Input: part model. Units: mm. Frame: model coordinates. A direction names the side the tool comes from. Coordinates: 2 decimals unless noted, no trailing zeros. Order: outer loops, then holes, each group sorted by start corner. A loop starts at its lowest first (then second) coordinate and runs counter-clockwise, first axis right, second up.
Autodesk Fusion 360 part; units mm, degrees
sketch "bottom" plane through (0, 0, 0) normal (0, 0, 1) x (1, 0, 0)
  line L0 (-22.5627, 0) -> (-67, 0)
  line L1 (-67, 88) -> (-22.5147, 88)
  circle A0 centre (-36, 69) radius 5
  circle A1 centre (-36, 19) radius 5
  line L2 (13.411, 30.589) -> (-13.3703, 3.8076)
  line L3 (13.435, 57.435) -> (-13.3223, 84.1924)
  line L4 (-67, 88) -> (-80, 88)
  line L5 (-80, 0) -> (-67, 0)
  arc A2 (-13.3223, 84.1924) -> (-22.5147, 88) centre (-22.5147, 75) ccw
  arc A3 (12.6084, 29.7863) -> (13.435, 57.435) centre (0, 44) ccw
  arc A4 (-22.5627, 0) -> (-13.3703, 3.8076) centre (-22.5627, 13) ccw
  line L6 (-64, 49) -> (-60, 49)
  line L7 (-60, 49) -> (-60, 39)
  line L8 (-60, 39) -> (-64, 39)
  circle A5 centre (-86, 44) radius 9.5
  line L9 (-64, 60) -> (-64, 49)
  line L10 (-64, 39) -> (-64, 28)
  arc A6 (-86, 63) -> (-85.9962, 25) centre (-86, 44) ccw
  line L11 (-67, 0) -> (-67, 25)
  line L12 (-67, 63) -> (-67, 88)
  line L13 (-67, 0) -> (-67, 25)
  line L14 (-67, 63) -> (-67, 88)
  arc A7 (-64, 28) -> (-67, 25) centre (-64, 25) ccw
  arc A8 (-67, 63) -> (-64, 60) centre (-64, 63) ccw
  line L15 (-85.9962, 25) -> (-86.0038, 25) construction
  arc A9 (-80, 19) -> (-86, 25) centre (-86, 19) ccw
  line L16 (-80, 19) -> (-80, 0)
  line L17 (-80, 88) -> (-80, 69)
  arc A10 (-86, 63) -> (-80, 69) centre (-86, 69) ccw
  dimension "d1" = 67
  dimension "d3" = 19
  dimension "d4" = 19
  dimension "d5" = 10
  dimension "d6" = 10
  dimension "d15" = 45
  dimension "d16" = 13
  dimension "d17" = 13
  dimension "d18" = 13
  dimension "d20" = 3
  dimension "d21" = 38
  dimension "d23" = 4
  dimension "d24" = 10
  dimension "d25" = 39
  dimension "d26" = 6
  dimension "d27" = 6
  dimension "d30" = 19
  dimension "d31" = 38
  dimension "d38" = 6
  dimension "d39" = 6
extrude "Extrude1" add sketch "bottom" along normal blind 10
extrude "Extrude2" cut sketch "bottom" along normal blind 40 contours L4 L5 L6 L7 L8 L9 L10 A6 L11 L12 L13 L14 A7 A8 A9 L16 L17 A10
extrude "Extrude3" add sketch "bottom" along normal blind 40 contours L4 L5 L6 L7 L8 L9 L10 A6 L11 L12 L13 L14 A7 A8 A9 L16 L17 A10
extrude "Extrude4" add 1 faces at (-71.3333, 73.3333, 40) along direction (0, 0, 1) blind 10
sketch "triangle" plane through (0, 0, 0) normal (0, -1, 0) x (1, 0, 0)
  line L0 (-80, 0) -> (-22.5627, 0)
  line L1 (-22.5627, 0) -> (-22.5627, 10)
  line L2 (-22.5627, 10) -> (-67, 10)
  line L3 (-67, 10) -> (-67, 50)
  line L4 (-67, 50) -> (-80, 50)
  line L5 (-80, 50) -> (-80, 0)
  line L6 (-60, 10) -> (-3, 10)
  line L7 (-60, 10) -> (-60, 50)
  line L8 (-60, 50) -> (-3, 10)
  dimension "d42" = 57
extrude "Extrude5" add sketch "triangle" along normal blind -49 and the other way blind 39 contours L2 L6 L7 L8
Item 1: Access query for faces 4 (the face through (-81.803, 23.288, 24.65)), 5 (the face through (-80, 79, 25)), 6 (the face through (-66.1, 60.86, 29.72)), 7 (the face through (-34, 54, 10)), 8 (the face through (-66.14, 27.1, 29.72)). Directions: +Z, -Z, +X, -X, +Y, -Y. A direction counts if a zero-diameter tool reaches every point of the face in a straight line with its end or side. Return the directions, or none.
Response values:
face 4: +Z, -Z, -X, -Y
face 5: +Z, -Z, -X, +Y
face 6: +Z, +X, +Y
face 7: +Z, +X
face 8: +Z, +X, -Y
Item 2: Cut plane C-C on z = 37. Return loops of the section in (x, y) (3 decimals), then the cut area to 3 significant figures.
Response values:
outline: (-86, 63) arc R19 ccw to (-85.996, 25) arc R6 cw to (-80, 19) - (-80, 0) - (-67, 0) - (-67, 25) arc R3 cw to (-64, 28) - (-64, 39) - (-41.475, 39) - (-41.475, 49) - (-64, 49) - (-64, 60) arc R3 cw to (-67, 63) - (-67, 88) - (-80, 88) - (-80, 69) arc R6 cw to start; hole circle Ø19 at (-86, 44)
area: 2,000 mm2
Item 3: Ray query, probe 1 along Y at (x, z) = (-36, 6.5); probe 2 along Y at (x, z) = (-59.5, 14); probe 3 along Y at (x, z) = (-86, 10.5). Return the intervals inside material, ascending.
Response values:
probe 1: y = 0 to 14, 24 to 64, 74 to 88
probe 2: y = 39 to 49
probe 3: y = 25 to 34.5, 53.5 to 63
Item 4: Draft query along X for faces 1 (the face through (-40, 66, 5)), 2 (the face through (-73, 45, 50)), 3 (the face through (-31.9, 43.93, 30.28)). Return one class per face: pulls with the +X half, pulls with the -X half, needs draft (parallel to the pull), parting line crosses it, or undercut.
Response values:
face 1: undercut
face 2: needs draft
face 3: pulls with the +X half
Item 5: Cut plane B-B on z = 8.5. Return loops of the section in (x, y) (3 decimals).
Response values:
outline: (-86, 63) arc R19 ccw to (-85.996, 25) arc R6 cw to (-80, 19) - (-80, 0) - (-22.563, 0) arc R13 ccw to (-13.37, 3.808) - (12.608, 29.786) arc R19 ccw to (13.435, 57.435) - (-13.322, 84.192) arc R13 ccw to (-22.515, 88) - (-80, 88) - (-80, 69) arc R6 cw to start; hole circle Ø19 at (-86, 44); hole circle Ø10 at (-36, 19); hole circle Ø10 at (-36, 69)
Item 6: Cut plane A-A on y = 44. Return loops of the section in (x, z).
Response values:
outline: (-105, 0) - (-95.5, 0) - (-95.5, 50) - (-105, 50) - close; (-76.5, 0) - (19, 0) - (19, 10) - (-3, 10) - (-60, 50) - (-76.5, 50) - close
Item 7: Cut plane D-D on x = 1.5. Return loops of the section in (y, z), then the cut area to 3 significant figures.
Response values:
outline: (18.68, 0) - (69.37, 0) - (69.37, 10) - (18.68, 10) - close
area: 507 mm2
Item 8: Pin query (flat end, axial travel): pin 1 Ø2 at (y, z) = (43, 40.5) entering from +X; pin 2 Ø7.5 at (y, z) = (13.5, 39) entering from +X; pin 3 Ø10 at (y, z) = (40.5, 30) entering from +X (3 decimals). Return the tip coordinate at first contact, or that it passes through.
Response values:
pin 1: stops at x = -45.04
pin 2: stops at x = -67
pin 3: stops at x = -24.375
